from build123d import *

# Parameters (mm, degrees)
SKETCH_1_W      = 40
SKETCH_1_H      = 64
SKETCH_1_R      = 1.6
SKETCH_1_R_2    = 1.1
EXTRUDE_1_DEPTH = 4
SKETCH_2_R      = 2.5
SKETCH_2_R_2    = 1.1
EXTRUDE_2_DEPTH = 2


with BuildPart() as part:
    # Эскиз1 → Бобышка-Вытянуть1 (new body)
    with BuildSketch(Plane.XY):
        Rectangle(SKETCH_1_W, SKETCH_1_H)
        with Locations((-13.25, 29)):
            Circle(SKETCH_1_R, mode=Mode.SUBTRACT)
        with Locations((13.25, 29)):
            Circle(SKETCH_1_R, mode=Mode.SUBTRACT)
        with Locations((-13.25, -29)):
            Circle(SKETCH_1_R, mode=Mode.SUBTRACT)
        with Locations((13.25, -29)):
            Circle(SKETCH_1_R, mode=Mode.SUBTRACT)
        with Locations((0, -21)):
            Circle(SKETCH_1_R_2, mode=Mode.SUBTRACT)
        with Locations((0, 17)):
            Circle(SKETCH_1_R_2, mode=Mode.SUBTRACT)
    extrude(amount=EXTRUDE_1_DEPTH)

    # Эскиз2 → Бобышка-Вытянуть2 (add)
    # profile 1 of 2: a face of its own
    with BuildSketch(Plane.XY.offset(4)):
        with Locations(Location((0, 17, 0), (0, 0, 180))):
            Circle(SKETCH_2_R)
        with Locations((0, 17)):
            Circle(SKETCH_2_R_2, mode=Mode.SUBTRACT)
    # profile 2 of 2: a face of its own
    with BuildSketch(Plane.XY.offset(4)):
        with Locations(Location((0, -21, 0), (0, 0, 180))):
            Circle(SKETCH_2_R)
        with Locations((0, -21)):
            Circle(SKETCH_2_R_2, mode=Mode.SUBTRACT)
    extrude(amount=EXTRUDE_2_DEPTH)


solid = part.part
Verification items for the finished model (mm, model axes). A direction names the side the tool comes from. Coordinates: 2 decimals unless noted, no trailing zeros. Write each loop counter-clockwise with the first axis right and the second up, starting at its lowest first coordinate (ties: lowest second). Pieces come first, ordered by that corner, then holes. Notation, with made-up numbers: (-14.5, -34) - (23.5, -34) arc R20 cw to (23.5, -27) - close; hole circle Ø4 at (35, -38). An arc over 180 degrees is marked (long way). Answer as a JSON object with one key per item and string values.
(1) Cross-section at A-A on x = -13.25. Record the cut outline in (y, z), plus the area to 3 significant figures.
Report:
{"outline": "(-32, 0) - (-30.6, 0) - (-30.6, 4) - (-32, 4) - close; (-27.4, 0) - (27.4, 0) - (27.4, 4) - (-27.4, 4) - close; (30.6, 0) - (32, 0) - (32, 4) - (30.6, 4) - close", "area": "230 mm^2"}
(2) Thickness scan on line 1 along Y through (x, z) = (13.25, 2.9); line 2 along Y through (x, z) = (0, 1.7); line 3 along Z through (x, y) = (-6, 13). Record the ranges inside material, lowest first.
Report:
{"line 1": "-32 to -30.6, -27.4 to 27.4, 30.6 to 32", "line 2": "-32 to -22.1, -19.9 to 15.9, 18.1 to 32", "line 3": "0 to 4"}
(3) Cross-section at D-D on y = 17. Record the cut outline in (x, z), plus the area to 3 significant figures.
Report:
{"outline": "(-20, 0) - (-1.1, 0) - (-1.1, 6) - (-2.5, 6) - (-2.5, 4) - (-20, 4) - close; (1.1, 0) - (20, 0) - (20, 4) - (2.5, 4) - (2.5, 6) - (1.1, 6) - close", "area": "157 mm^2"}
(4) Cross-section at B-B on z = 2.85. Record the cut outline in (x, y), plus the area to 3 significant figures.
Report:
{"outline": "(-20, -32) - (20, -32) - (20, 32) - (-20, 32) - close; hole circle Ø3.2 at (-13.25, -29); hole circle Ø3.2 at (-13.25, 29); hole circle Ø2.2 at (0, -21); hole circle Ø2.2 at (0, 17); hole circle Ø3.2 at (13.25, -29); hole circle Ø3.2 at (13.25, 29)", "area": "2,520 mm^2"}
(5) Mould release check, pull along X, two halves, no side actions. Record for faces 1 (the cylindrical face through (12, -28, 2)), 2 (the flat face through (20, 0, 2)), 3 (the flat face through (0, 32, 2)), 4 (the cylindrical face through (-14.43, 30.08, 1.97)): pulls with the +X half, pulls with the -X half, needs draft (parallel to the pull), parting line crosses it, or undercut.
Report:
{"face 1": "undercut", "face 2": "pulls with the +X half", "face 3": "needs draft", "face 4": "undercut"}
(6) Gauge pin test, flat ends, axial feed: pin 1 Ø3 at (x, y) = (-13.25, 29) entering from -Z; pin 2 Ø10 at (x, y) = (-10.5, 3.5) entering from +Z. Record the tip position at first contact, or that the pin passes through.
Report:
{"pin 1": "through", "pin 2": "z = 4"}
(7) Cross-section at C-C on y = -29. Record the cut outline in (x, z), plus the area to 3 significant figures.
Report:
{"outline": "(-20, 0) - (-14.85, 0) - (-14.85, 4) - (-20, 4) - close; (-11.65, 0) - (11.65, 0) - (11.65, 4) - (-11.65, 4) - close; (14.85, 0) - (20, 0) - (20, 4) - (14.85, 4) - close", "area": "134 mm^2"}
(8) Tool access check on faces 5 (the cylindrical face through (0.33, -23.48, 4.99)), 6 (the cylindrical face through (-0.238, 15.926, 2.958)). Record the directions out of +Z, -Z, +X, -X, +Y, -Y that give a thin tool (end or side, any length) a straight path to the whole face; none if there is none.
Report:
{"face 5": "+Z", "face 6": "+Z, -Z"}
